Check sheet for the modelled part. Datum: model origin and axes. Units: mm. A direction names the side the tool comes from. Coordinates: 2 decimals unless noted, no trailing zeros. Write each loop counter-clockwise with the first axis right and the second up, starting at its lowest first coordinate (ties: lowest second). Pieces come first, ordered by that corner, then holes. Notation, with made-up numbers: (-12.75, 74) -> (44.25, 74) arc R26 cw to (44.25, 101) -> close; hole circle Ø4 at (-28, 45). An arc over 180 degrees is marked (long way). One line per item, written item: value. Start each with the question number.
1) Draft check along X on faces 1 (the flat face through (156, 0.1, -7)), 2 (the cylindrical face through (156.38, 4.51, -7.68)), 3 (the cylindrical face through (161.794, 3.096, -6.634)), 4 (the flat face through (154.9, 6, -7)). Enter one of: +X half, -X half, draft (parallel to the pull), parting line (faces both ways), or undercut.
2) Sectioned sample at D-D on x = 154. Enter the section's corners in (y, z).
3) Scan lines: line 1 along X through (y, z) = (36.5, -5.25); line 2 along Y through (x, z) = (158, -6.75); line 3 along Y through (x, z) = (159, -12.25). Record each from-to range of solid material in increasing order. Write a range as [from, to].
4) Sectioned sample at C-C on y = 22.5. Enter the section's corners in (x, z).
5) Sectioned sample at B-B on z = -9.5. Enter the section's corners in (x, y) (3 decimals), plus the area to 3 significant figures.
6) Gauge pin test, flat ends, axial feed: P1, Ø6, axis at y = 8, z = -6, coming from the -X side; P2, Ø1.2, axis at y = 18, z = 0.5, coming from the +X side; P3, Ø4, axis at x = 158.5, y = 18, coming from the -Z side; P4, Ø0.9, axis at x = 153.5, y = 13, coming from the -Z side. Record the tip position at first contact, or that the pin passes through.
7) Sectioned sample at A-A on y = 4. Enter the section's corners in (x, z), plus the area to 3 significant figures.
8) Set-up check for faces 5 (the flat face through (154.9, 34, -7)), 6 (the flat face through (154, 20, 1.5)), 7 (the cylindrical face through (156.749, 30.743, -6.634)): record each of +Z, -Z, +X, -X, +Y, -Y from which the full face is reachable in a straight line by a thin tool's end or side.
```python
from build123d import *

# Parameters (mm, degrees)
SKETCH_1_W                  = 155
SKETCH_1_H                  = 40.5
EXTRUDE_1_DEPTH             = 1.5
EXTRUDE_2_DEPTH             = 1.5
FILLET_2_R                  = 8
CUT_EXTRUDE_1_DEPTH         = 167.992514924
SKETCH_5_W                  = 152.3
SKETCH_5_H                  = 40.3
CUT_EXTRUDE_2_DEPTH         = 167.871267749
EXTRUDE_3_DEPTH             = 15
FILLET_START                = -16
FILLET_3_DEPTH              = 16
HOLE_WIZARD_M31_D           = 3.4
HOLE_WIZARD_M31_CSINK_D     = 6.72
HOLE_WIZARD_M31_CSINK_ANGLE = 90


with BuildPart() as part:
    # Эскиз1 → Бобышка-Вытянуть1 (new body)
    with BuildSketch(Plane.XY):
        with Locations((77.5, 20.25)):
            Rectangle(SKETCH_1_W, SKETCH_1_H)
    extrude(amount=EXTRUDE_1_DEPTH)

    # Эскиз2 → Бобышка-Вытянуть2 (add)
    with BuildSketch(Plane(origin=(0, 0, 0), x_dir=(-1, 0, 0), z_dir=(0, 0, -1))):
        with BuildLine():
            Line((-158, 0), (-155, 0))
            Line((-155, 0), (-155, 8))
            Line((-155, 8), (-158, 8))
            ThreePointArc((-158, 8), (-162, 4), (-158, 0))
        make_face()
        with BuildLine():
            Line((-155, 32.5), (-155, 40.5))
            Line((-155, 40.5), (-158, 40.5))
            ThreePointArc((-158, 40.5), (-162, 36.5), (-158, 32.5))
            Line((-158, 32.5), (-155, 32.5))
        make_face()
    extrude(amount=-EXTRUDE_2_DEPTH)

    # Скругление2
    fillet_2_edges = [part.edges().sort_by_distance(p)[0] for p in [
        (155, 8, 0.75),
        (155, 32.5, 0.75),
    ]]
    fillet(fillet_2_edges, radius=FILLET_2_R)

    # Эскиз3 → Вырез-Вытянуть1 (cut, through all)
    with BuildSketch(Plane.XY.offset(1.5)):
        with BuildLine():
            Line((155, 14.908712115), (155, 25.591287885))
            ThreePointArc((155, 25.591287885), (156.266996708, 29.911781684), (159.666666667, 32.863762628))
            ThreePointArc((159.666666667, 32.863762628), (161.908001374, 37.352950911), (158, 40.5))
            Line((158, 40.5), (0, 40.5))
            Line((0, 40.5), (0, 0))
            Line((0, 0), (158, 0))
            ThreePointArc((158, 0), (161.908001374, 3.147049089), (159.666666667, 7.636237372))
            ThreePointArc((159.666666667, 7.636237372), (156.266996708, 10.588218316), (155, 14.908712115))
        make_face()
        with BuildLine():
            Line((154.9, 14.908712115), (154.9, 25.591287885))
            ThreePointArc((154.9, 25.591287885), (156.182834167, 29.965787857), (159.625, 32.954668563))
            ThreePointArc((159.625, 32.954668563), (161.81030134, 37.331627138), (158, 40.4))
            Line((158, 40.4), (0.1, 40.4))
            Line((0.1, 40.4), (0.1, 0.1))
            Line((0.1, 0.1), (158, 0.1))
            ThreePointArc((158, 0.1), (161.81030134, 3.168372862), (159.625, 7.545331437))
            ThreePointArc((159.625, 7.545331437), (156.182834167, 10.534212143), (154.9, 14.908712115))
        make_face(mode=Mode.SUBTRACT)
    extrude(amount=-CUT_EXTRUDE_1_DEPTH, mode=Mode.SUBTRACT)

    # Эскиз5 → Вырез-Вытянуть2 (cut, through all)
    with BuildSketch(Plane(origin=(0, 0, 0), x_dir=(-1, 0, 0), z_dir=(0, 0, -1))):
        with Locations((-76.25, 20.25)):
            Rectangle(SKETCH_5_W, SKETCH_5_H)
    extrude(amount=-CUT_EXTRUDE_2_DEPTH, mode=Mode.SUBTRACT)

    # Эскиз6 → Бобышка-Вытянуть3 (add)
    with BuildSketch(Plane(origin=(0, 0, 0), x_dir=(-1, 0, 0), z_dir=(0, 0, -1))):
        with BuildLine():
            Line((-154.9, 40.4), (-154.9, 25.591287885))
            ThreePointArc((-154.9, 25.591287885), (-156.182834167, 29.965787857), (-159.625, 32.954668563))
            ThreePointArc((-159.625, 32.954668563), (-161.81030134, 37.331627138), (-158, 40.4))
            Line((-158, 40.4), (-154.9, 40.4))
        make_face()
        with BuildLine():
            Line((-154.9, 0.1), (-154.9, 14.908712115))
            ThreePointArc((-154.9, 14.908712115), (-156.182834167, 10.534212143), (-159.625, 7.545331437))
            ThreePointArc((-159.625, 7.545331437), (-161.81030134, 3.168372862), (-158, 0.1))
            Line((-158, 0.1), (-154.9, 0.1))
        make_face()
    extrude(amount=EXTRUDE_3_DEPTH)

    # Скругление3: read off the stored shape, not the designer's step
    # Скругление3 outline → Скругление3 (cut)
    with BuildSketch(Plane.XY.offset(FILLET_START)):
        with BuildLine():
            ThreePointArc((154.9, 12.363127702), (155.068953979, 12.56070337), (155.290361446, 12.424467086))
            ThreePointArc((155.290361446, 12.424467086), (154.998185447, 13.651348263), (154.9, 14.908712115))
            Line((154.9, 14.908712115), (154.9, 12.363127702))
        make_face()
        with BuildLine():
            ThreePointArc((155.290361446, 28.075532914), (155.068953979, 27.93929663), (154.9, 28.136872298))
            Line((154.9, 28.136872298), (154.9, 25.591287885))
            ThreePointArc((154.9, 25.591287885), (154.998185447, 26.848651737), (155.290361446, 28.075532914))
        make_face()
    extrude(amount=FILLET_3_DEPTH, mode=Mode.SUBTRACT)

    # Зенковка для  винта с потайной головкой с внутренним шестигранником M31 (through all)
    with Locations(Plane.XY.offset(1.5)):
        with Locations((158, 36.5), (158, 4)):
            CounterSinkHole(HOLE_WIZARD_M31_D / 2, HOLE_WIZARD_M31_CSINK_D / 2, counter_sink_angle=HOLE_WIZARD_M31_CSINK_ANGLE)


solid = part.part
```
Answers:
1. face 1: draft
1. face 2: undercut
1. face 3: +X half
1. face 4: -X half
2. outline: (0.1, 0) -> (40.4, 0) -> (40.4, 1.5) -> (0.1, 1.5) -> close
3. line 1: x = [154.9, 156.3], [159.7, 161.9]
3. line 2: y = [0.1, 2.3], [5.7, 8.54], [31.96, 34.8], [38.2, 40.4]
3. line 3: y = [0.23, 2.63], [5.37, 7.87], [32.63, 35.13], [37.87, 40.27]
4. outline: (152.4, 0) -> (154.9, 0) -> (154.9, 1.5) -> (152.4, 1.5) -> close
5. outline: (154.9, 0.1) -> (158, 0.1) arc R3.9 ccw to (159.625, 7.545) arc R8.1 cw to (155.29, 12.424) arc R0.2 ccw to (154.9, 12.363) -> close; (154.9, 28.137) arc R0.2 ccw to (155.29, 28.076) arc R8.1 cw to (159.625, 32.955) arc R3.9 ccw to (158, 40.4) -> (154.9, 40.4) -> close; hole circle Ø3.4 at (158, 4); hole circle Ø3.4 at (158, 36.5)
5. area: 94.0 mm2
6. P1: stops at x = 154.9
6. P2: stops at x = 154.9
6. P3: passes through
6. P4: stops at z = 0
7. outline: (152.4, 0) -> (154.9, 0) -> (154.9, -15) -> (156.3, -15) -> (156.3, -0.16) -> (154.64, 1.5) -> (152.4, 1.5) -> close; (159.7, -15) -> (161.9, -15) -> (161.9, 1.5) -> (161.36, 1.5) -> (159.7, -0.16) -> close
7. area: 60.4 mm2
8. face 5: -Z, -X, +Y, -Y
8. face 6: +Z, +X, -X, +Y, -Y
8. face 7: +Z, -Z, +X
